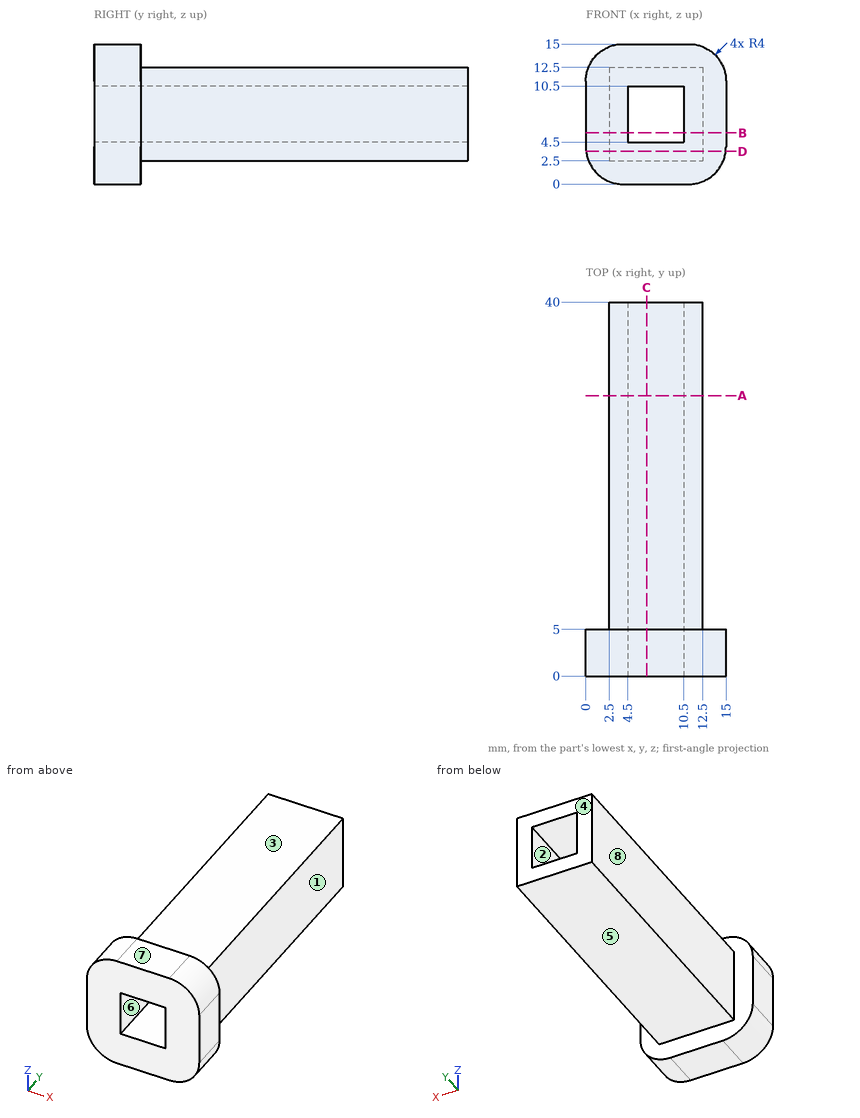
Geometry check sheet. Reference: drawing and pictorial views, mm from the part's lowest x, y, z. A direction names the side the tool comes from. Coordinates: 2 decimals unless noted, no trailing zeros. Order: outer loops, then holes, each group sorted by start corner. A loop starts at its lowest first (then second) coordinate and runs counter-clockwise, first axis right, second up. Notation, with made-up numbers: M -19,14.25 L -3,14.25 A13 ccw -3,32.25 Z; hole C -14,80.5 d4. An arc over 180 degrees is marked long. Write each question's results on one line, items separated by ' | '. Start each with the question number.
1. Access from +Z, -Z, +X, -X, +Y, -Y to the whole of each face (thin tool, end or side, straight path). Record for the marked faces 1, 2, 3, 4 and 5.
2. Mould release check, pull along X, two halves, no side actions. Record for the marked faces 6, 7 and 8: +X half, -X half, draft (parallel to the pull), parting line (faces both ways), or undercut.
3. Cross-section at A-A on y = 30. Record the cut outline in (x, z).
4. Go/stop test with flat-tipped pins: P1, Ø3, axis at x = 9.5, y = 15, coming from the +Z side; P2, Ø1.8, axis at y = 12.5, z = 6.5, coming from the -X side; P3, Ø8, axis at x = 10.5, y = 20, coming from the -Z side. Record where each tip stops, or that it passes through.
5. Cross-section at D-D on z = 3.5. Record the cut outline in (x, y), and give its area (3 significant figures).
6. Cross-section at B-B on z = 5.5. Record the cut outline in (x, y).
7. Cross-section at C-C on x = 6.5. Record the cut outline in (y, z).
8. Material ranges on probe 1 along X at (y, z) = (37, 6.5); probe 2 along Y at (x, z) = (2.25, 4.5), recorded low to high.
Checks:
1) face 1: +Z, -Z, +X, +Y | face 2: +Y, -Y | face 3: +Z, +X, -X, +Y | face 4: +Z, -Z, +X, -X, +Y | face 5: -Z, +X, -X, +Y
2) face 6: undercut | face 7: draft | face 8: -X half
3) outline: M 2.5,2.5 L 12.5,2.5 L 12.5,12.5 L 2.5,12.5 Z; hole M 4.5,4.5 L 10.5,4.5 L 10.5,10.5 L 4.5,10.5 Z
4) P1: stops at z = 12.5 | P2: stops at x = 2.5 | P3: stops at z = 2.5
5) outline: M 0.03,0 L 14.97,0 L 14.97,5 L 12.5,5 L 12.5,40 L 2.5,40 L 2.5,5 L 0.03,5 Z | area: 425 mm²
6) outline: M 0,0 L 4.5,0 L 4.5,40 L 2.5,40 L 2.5,5 L 0,5 Z; M 10.5,0 L 15,0 L 15,5 L 12.5,5 L 12.5,40 L 10.5,40 Z
7) outline: M 0,0 L 5,0 L 5,2.5 L 40,2.5 L 40,4.5 L 0,4.5 Z; M 0,10.5 L 40,10.5 L 40,12.5 L 5,12.5 L 5,15 L 0,15 Z
8) probe 1: x = 2.5 to 4.5, 10.5 to 12.5 | probe 2: y = 0 to 5
